Can you work these out from the model? Positions are in its coordinate system, mm. A direction names the side the tool comes from. Coordinates: 2 decimals unless noted, no trailing zeros. Loops run counter-clockwise (first coordinate to the right, second up) from the corner with the lowest first, then second, coordinate; pieces in that order, holes last. Notation, with made-up numbers: (60.25, 43.5) -> (89.25, 43.5) arc R24 cw to (89.25, 80.5) -> close; hole circle Ø6 at (-16, 70.5). An arc over 180 degrees is marked (long way). Use one line per item in the form item = value. Start each with the question number.
(1) Imagine slicing it at B-B (x = -174). List the corners of the cut face in (y, z) for me, plus the area to 3 significant figures.
(2) Imagine slicing it at C-C (z = 30). List the corners of the cut face in (x, y) for me, plus the area to 3 significant figures.
(3) I need wall thicknesses on line 1 (Y direction, x = 50, z = -36); line 2 (Z direction, x = -29, y = 17); line 3 (Y direction, x = -57.5, z = 26). Which ranges of each line are inside material? Lowest first, please. Write a range as [from, to].
(4) Imagine slicing it at A-A (y = 20). List the corners of the cut face in (x, z) for me.
(5) Thinking about a two-plate mould opening in Z: for faces 3 (the flat face through (-3, 3, 0)), 4 (the flat face through (200, 2, 0)), 5 (the flat face through (-3, 12, -38)), which applies, released by +Z, released by -Z, zero draft, split by the parting line, or undercut?
(6) I'm going to push flat-ended pins straight in: pin 1 (3.5 mm diameter, centred on x = -150, y = 12.5, fed in from -Z); pin 2 (4 mm diameter, centred on x = 113, z = 18, fed in from +Y). Where does each tip first touch, or does it pass through?
(7) On a 3-axis mill with a long thin cutter (end or side, diameter ignored), from which of +Z, -Z, +X, -X, +Y, -Y can I reach the whole of each face in a straight line? I mean faces 1 (the flat face through (-3, 0, -1)), 2 (the flat face through (-3, 14, -35)). Say none if no direction works.
```python
from build123d import *

# Parameters (mm, degrees)
ESBO_O1_W                = 400
ESBO_O1_H                = 76
RESSALTO_EXTRUS_O1_DEPTH = 3
ESBO_O2_W                = 400
ESBO_O2_H                = 3
RESSALTO_EXTRUS_O2_DEPTH = 22
FURO_COM_FOLGA_DE_M41_D  = 4.5


with BuildPart() as part:
    # Esboço1 → Ressalto-extrusão1 (new body)
    with BuildSketch(Plane(origin=(0, 0, 0), x_dir=(1, 0, 0), z_dir=(0, 1, 0))):
        Rectangle(ESBO_O1_W, ESBO_O1_H)
    extrude(amount=RESSALTO_EXTRUS_O1_DEPTH)

    # Esboço2 → Ressalto-extrusão2 (add)
    with BuildSketch(Plane(origin=(0, 3, 0), x_dir=(1, 0, 0), z_dir=(0, 1, 0))):
        with Locations((0, 36.5)):
            Rectangle(ESBO_O2_W, ESBO_O2_H)
        with Locations((0, -36.5)):
            Rectangle(ESBO_O2_W, ESBO_O2_H)
    extrude(amount=RESSALTO_EXTRUS_O2_DEPTH)

    # Furo com folga de M41 (through all)
    with Locations(Plane(origin=(-150, 12.5, 38), x_dir=(1, 0, 0), z_dir=(0, 0, 1))):
        with Locations((0, 0), (300, 0), (100, 0), (200, 0)):
            Hole(FURO_COM_FOLGA_DE_M41_D / 2)


solid = part.part
```
Worked out:
q1.outline = (0, -38) -> (25, -38) -> (25, -35) -> (3, -35) -> (3, 35) -> (25, 35) -> (25, 38) -> (0, 38) -> close
q1.area = 360 mm2
q2.outline = (-200, 0) -> (200, 0) -> (200, 3) -> (-200, 3) -> close
q2.area = 1,200 mm2
q3.line_1 = [0, 10.25], [14.75, 25]
q3.line_2 = [-38, -35], [35, 38]
q3.line_3 = [0, 3]
q4.outline = (-200, -38) -> (200, -38) -> (200, -35) -> (-200, -35) -> close; (-200, 35) -> (200, 35) -> (200, 38) -> (-200, 38) -> close
q5.face_3 = undercut
q5.face_4 = zero draft
q5.face_5 = released by -Z
q6.pin_1 = through
q6.pin_2 = 3
q7.face_1 = +Z, -Z, +X, -X, -Y
q7.face_2 = +X, -X, +Y
